from build123d import *

# Parameters (mm, degrees)
EXTRUDE_1_DEPTH          = 2.5
EXTRUDE_1_DEPTH_BACK     = 2.5
SKETCH_1_R               = 2
EXTRUDE_2_DEPTH          = 3
SKETCH_4_W               = 5
SKETCH_4_H               = 21
EXTRUDE_3_DEPTH          = 1.8
CUT_EXTRUDE_1_DEPTH      = 72.103790411
CUT_EXTRUDE_1_DEPTH_BACK = 72.103790411
SHELL_START              = 62.288432405
SHELL_1_DEPTH            = 2
SHELL_START_2            = 63.288432405
SHELL_1_2_OUTLINE_W      = 1
SHELL_1_2_OUTLINE_H      = 12
SHELL_1_2_DEPTH          = 1
EXTRUDE_4_DEPTH          = 1
EXTRUDE_5_DEPTH          = 1.8


with BuildPart() as part:
    # 草图1 → 凸台-拉伸1 (new, two sides: drawn at the far end of the back side and taken through both)
    # profile 1 of 2: a face of its own
    with BuildSketch(Plane.XY.offset(-EXTRUDE_1_DEPTH_BACK)):
        with Locations((54.288432405, 0.720527774)):
            Circle(SKETCH_1_R)
    # profile 2 of 2: a face of its own
    with BuildSketch(Plane.XY.offset(-EXTRUDE_1_DEPTH_BACK)):
        Polygon((54.288432405, 0.720527774), (62.288432405, 0.720527774), (62.288432405, -13.279472226), (62.288432405, -21.279472226), (54.288432405, -13.279472226), align=None)
        Polygon((56.288432405, -12.451045101), (60.288432405, -16.451045101), (60.288432405, -13.279472226), (60.288432405, -1.279472226), (56.288432405, -5.279472226), align=None, mode=Mode.SUBTRACT)
    extrude(amount=EXTRUDE_1_DEPTH + EXTRUDE_1_DEPTH_BACK)

    # 草图2 → 凸台-拉伸2 (add)
    with BuildSketch(Plane(origin=(62.288432405, 0, 0), x_dir=(0, 0, -1), z_dir=(1, 0, 0))):
        Polygon((-7, -3.279472226), (-4.5, -27.279472226), (4.5, -27.279472226), (7, -3.279472226), (7, 8.720527774), (-7, 8.720527774), align=None)
    extrude(amount=EXTRUDE_2_DEPTH)

    # 草图4 → 凸台-拉伸3 (add)
    with BuildSketch(Plane.ZY.offset(-62.288432405)):
        Polygon((-2.5, -0.279472226), (-7, -0.279472226), (-7, -3.279472226), (-4.5, -27.279472226), (4.5, -27.279472226), (7, -3.279472226), (7, -0.279472226), (2.5, -0.279472226), (2.5, -21.279472226), (-2.5, -21.279472226), align=None)
        with Locations((0, -10.779472226)):
            Rectangle(SKETCH_4_W, SKETCH_4_H)
    extrude(amount=EXTRUDE_3_DEPTH)

    # 草图5 → 切除-拉伸1 (cut, two sides: drawn at the far end of the back side and taken through both)
    with BuildSketch(Plane.XY.offset(-CUT_EXTRUDE_1_DEPTH_BACK)):
        Polygon((47.883968073, 6.720527774), (47.883968073, -27.279472226), (62.288432405, -27.279472226), (62.288432405, -3.279472226), (63.288432405, -2.279472226), (63.288432405, 6.720527774), (62.288432405, 6.720527774), align=None)
    extrude(amount=CUT_EXTRUDE_1_DEPTH + CUT_EXTRUDE_1_DEPTH_BACK, mode=Mode.SUBTRACT)

    # 抽壳1: read off the stored shape, not the designer's step
    # 抽壳1 outline → 抽壳1 (cut)
    with BuildSketch(Plane.YZ.offset(SHELL_START)):
        Polygon((6.720527774, -6), (6.720527774, 6), (-3.227529416, 6), (-26.279472226, 3.598755957), (-26.279472226, -3.598755957), (-3.227529416, -6), align=None)
    extrude(amount=SHELL_1_DEPTH, mode=Mode.SUBTRACT)

    # Shell 1 2 outline → Shell 1 2 (cut)
    with BuildSketch(Plane.YZ.offset(SHELL_START_2)):
        with Locations((7.220527774, 0)):
            Rectangle(SHELL_1_2_OUTLINE_W, SHELL_1_2_OUTLINE_H)
    extrude(amount=SHELL_1_2_DEPTH, mode=Mode.SUBTRACT)

    # 草图7 → 凸台-拉伸4 (add)
    with BuildSketch(Plane.ZY.offset(-63.288432405)):
        Polygon((-6, 4.720527774), (-6, 6.720527774), (-7, 6.720527774), (-7, 0.720527774), align=None)
        Polygon((6, 4.720527774), (7, 0.720527774), (7, 6.720527774), (6, 6.720527774), align=None)
    extrude(amount=EXTRUDE_4_DEPTH)

    # 草图6 → 凸台-拉伸5 (add)
    with BuildSketch(Plane.ZY.offset(-62.288432405)):
        Polygon((3.598755957, -26.279472226), (5.890422624, -4.279472226), (7, -3.279472226), (4.5, -27.279472226), (-4.5, -27.279472226), (-7, -3.279472226), (-5.890422624, -4.279472226), (-3.598755957, -26.279472226), align=None)
    extrude(amount=EXTRUDE_5_DEPTH)


solid = part.part
Check sheet for the modelled part. Datum: model origin and axes. Units: mm. A direction names the side the tool comes from. Give positions to 0.01 mm unless a question says otherwise; leave off trailing zeros. Loops run counter-clockwise (first coordinate to the right, second up) from the corner with the lowest first, then second, coordinate; pieces in that order, holes last. Notation, with made-up numbers: M -40,81.5 L -4,81.5 A5 cw -4,89.5 Z; hole C -5.75,80.5 d1. An arc over 180 degrees is marked long. Return JSON: item names as keys, results as strings. Group by question number.
1. Thickness scan on L1, parallel to Y at x = 63.9, z = 1.75; L2, parallel to X at y = 7.5, z = -3.25; L3, parallel to X at y = -3, z = 0. Record the ranges inside material, lowest first.
2. Cross-section at B-B on x = 62.85. Record the boundary of the cut face in (y, z), plus the area to 3 significant figures.
3. Cross-section at C-C on z = 3.25. Record the boundary of the cut face in (x, y), plus the area to 3 significant figures.
4. Cross-section at D-D on y = -1. Record the boundary of the cut face in (x, z).
5. Mould release check, pull along Z, two halves, no side actions. Record for faces 4 (the flat face through (64, 3, 7)), 5 (the flat face through (64, 3, -7)), 6 (the flat face through (63, -27.279, 0)), 7 (the flat face through (63, 6.721, 0)): released by +Z, released by -Z, zero draft, split by the parting line, or undercut.
6. Cross-section at A-A on y = 6. Record the boundary of the cut face in (x, z), plus the area to 3 significant figures.
7. Go/stop test with flat-tipped pins: pin 1 (1.5 mm diameter, centred on y = -6, z = -2, fed in from -X); pin 2 (1.1 mm diameter, centred on y = 1, z = 6.5, fed in from -X); pin 3 (2 mm diameter, centred on x = 61, y = -21.5, fed in from -Z). Record where each tip stops, or that it passes through.
8. Tool access check on faces 1 (the flat face through (62.288, 7, 0)), 2 (the flat face through (62.288, -3.6, 6.3)), 3 (the flat face through (62.795, 2.693, -6.507)). Record the directions out of +Z, -Z, +X, -X, +Y, -Y that give a thin tool (end or side, any length) a straight path to the whole face; none if there is none.
Return value:
{
 "1": {"L1": "-27.28 to -26.28, 7.72 to 8.72", "L2": "62.29 to 63.29, 64.29 to 65.29", "L3": "64.29 to 65.29"},
 "2": {"outline": "M -27.28,-4.5 L -3.28,-7 L -2.72,-7 L -2.72,-6 L -3.23,-6 L -26.28,-3.6 L -26.28,3.6 L -3.23,6 L -2.72,6 L -2.72,7 L -3.28,7 L -27.28,4.5 Z; M 0.72,-7 L 8.72,-7 L 8.72,7 L 0.72,7 L 4.72,6 L 6.72,6 L 6.72,-6 L 4.72,-6 Z", "area": "92.5 mm^2"},
 "3": {"outline": "M 60.49,-27.28 L 65.29,-27.28 L 65.29,8.72 L 62.29,8.72 L 62.29,6.72 L 63.29,6.72 L 63.29,7.72 L 64.29,7.72 L 64.29,-26.28 L 60.49,-26.28 Z", "area": "42.8 mm^2"},
 "4": {"outline": "M 63.29,-7 L 65.29,-7 L 65.29,7 L 63.29,7 L 63.29,6 L 64.29,6 L 64.29,-6 L 63.29,-6 Z"},
 "5": {"face 4": "released by +Z", "face 5": "released by -Z", "face 6": "zero draft", "face 7": "undercut"},
 "6": {"outline": "M 62.29,-7 L 65.29,-7 L 65.29,7 L 62.29,7 L 62.29,6 L 64.29,6 L 64.29,-6 L 62.29,-6 Z", "area": "18.0 mm^2"},
 "7": {"pin 1": "x = 64.29", "pin 2": "x = 62.29", "pin 3": "z = -5.21"},
 "8": {"face 1": "+Z, -Z, -X, +Y", "face 2": "-X, +Y", "face 3": "-X"}
}
